from build123d import *

# Parameters (mm, degrees)
SKETCH1_W                                            = 150
SKETCH1_H                                            = 300
BOSS_EXTRUDE1_DEPTH                                  = 20
SKETCH2_W                                            = 150
SKETCH2_H                                            = 8
BOSS_EXTRUDE2_DEPTH                                  = 3
CBORE_FOR_M6_HEX_SOCKET_THIN_HEAD_CAP_SC_D           = 6.6
CBORE_FOR_M6_HEX_SOCKET_THIN_HEAD_CAP_SC_DEPTH       = 24.5
CBORE_FOR_M6_HEX_SOCKET_THIN_HEAD_CAP_SC_CBORE_D     = 11
CBORE_FOR_M6_HEX_SOCKET_THIN_HEAD_CAP_SC_CBORE_DEPTH = 4.5
M8_TAPPED_HOLE1_D                                    = 6.8
M8_TAPPED_HOLE1_DEPTH                                = 33.75
FILLET1_R                                            = 2.5


with BuildPart() as part:
    # Sketch1 → Boss-Extrude1 (new body)
    with BuildSketch(Plane(origin=(0, 0, 0), x_dir=(1, 0, 0), z_dir=(0, 1, 0))):
        Rectangle(SKETCH1_W, SKETCH1_H)
    extrude(amount=BOSS_EXTRUDE1_DEPTH)

    # Sketch2 → Boss-Extrude2 (add)
    with BuildSketch(Plane(origin=(0, 0, 0), x_dir=(1, 0, 0), z_dir=(0, 1, 0))):
        with Locations((0, -130)):
            Rectangle(SKETCH2_W, SKETCH2_H)
        with Locations((0, 130)):
            Rectangle(SKETCH2_W, SKETCH2_H)
    extrude(amount=-BOSS_EXTRUDE2_DEPTH)

    # CBORE for M6 Hex Socket Thin Head Cap Screw1
    with Locations(Plane(origin=(0, 20, 0), x_dir=(1, 0, 0), z_dir=(0, 1, 0))):
        with Locations((0, -130), (0, 130)):
            CounterBoreHole(CBORE_FOR_M6_HEX_SOCKET_THIN_HEAD_CAP_SC_D / 2, CBORE_FOR_M6_HEX_SOCKET_THIN_HEAD_CAP_SC_CBORE_D / 2, CBORE_FOR_M6_HEX_SOCKET_THIN_HEAD_CAP_SC_CBORE_DEPTH, depth=CBORE_FOR_M6_HEX_SOCKET_THIN_HEAD_CAP_SC_DEPTH)

    # M8 Tapped Hole1
    with Locations(Plane.ZY.offset(75)):
        with Locations((0, 10)):
            Hole(M8_TAPPED_HOLE1_D / 2, depth=M8_TAPPED_HOLE1_DEPTH)

    # Fillet1
    fillet1_edges = [part.edges().sort_by_distance(p)[0] for p in [
        (-75, 10, -150),
        (75, 10, -150),
        (75, 10, 150),
        (-75, 10, 150),
    ]]
    fillet(fillet1_edges, radius=FILLET1_R)


solid = part.part
Geometry check sheet. Reference: the model listing, model coordinates, mm. A direction names the side the tool comes from. Give positions to 0.01 mm unless a question says otherwise; leave off trailing zeros. Order: outer loops, then holes, each group sorted by start corner. A loop starts at its lowest first (then second) coordinate and runs counter-clockwise, first axis right, second up. Notation, with made-up numbers: (14.5, -2.5) - (69.5, -2.5) arc R20 ccw to (69.5, 27.5) - close; hole circle Ø2 at (11.5, 85). An arc over 180 degrees is marked (long way). Answer as a JSON object with one key per item and string values.
(1) Cross-section at B-B (z = 130). Record the cut outline in (x, y), then the cut area to 3 significant figures.
Report:
{"outline": "(-75, -3) - (-3.3, -3) - (-3.3, 15.5) - (-5.5, 15.5) - (-5.5, 20) - (-75, 20) - close; (3.3, -3) - (75, -3) - (75, 20) - (5.5, 20) - (5.5, 15.5) - (3.3, 15.5) - close", "area": "3,280 mm^2"}
(2) Cross-section at D-D (z = -36.5). Record the cut outline in (x, y).
Report:
{"outline": "(-75, 0) - (75, 0) - (75, 20) - (-75, 20) - close"}
(3) Depth check by flat-ended pin: pin 1 Ø5 at (x, z) = (-59.5, -109) entering from -Y; pin 2 Ø0.9 at (x, y) = (33.5, -1) entering from -Z; pin 3 Ø2 at (y, z) = (10, -0.5) entering from -X. Enter the tip coordinate at first touch or a pass-through.
Report:
{"pin 1": "y = 0", "pin 2": "z = -134", "pin 3": "x = -41.25"}
(4) Material ranges on line 1 (Z direction, x = 0, y = 6.5); line 2 (Y direction, x = -59, z = 0); line 3 (X direction, y = 18.15, z = 130), recorded low to high.
Report:
{"line 1": "-150 to -133.3, -126.7 to 126.7, 133.3 to 150", "line 2": "0 to 6.6, 13.4 to 20", "line 3": "-75 to -5.5, 5.5 to 75"}
(5) Tool access check on faces 5 (the flat face through (-1, 0, -2)), 6 (the flat face through (-1, 0, -142)), 7 (the flat face through (-1, 0, 142)), 8 (the flat face through (0, 15.5, 134)), 9 (the cylindrical face through (-57.89, 6.68, 0.74)). Record the directions out of +Z, -Z, +X, -X, +Y, -Y that give a thin tool (end or side, any length) a straight path to the whole face; none if there is none.
Report:
{"face 5": "+X, -X, -Y", "face 6": "-Z, +X, -X, -Y", "face 7": "+Z, +X, -X, -Y", "face 8": "+Y", "face 9": "-X"}
(6) Cross-section at C-C (z = 0). Record the cut outline in (x, y).
Report:
{"outline": "(-75, 0) - (75, 0) - (75, 20) - (-75, 20) - (-75, 13.4) - (-41.25, 13.4) - (-41.25, 6.6) - (-75, 6.6) - close"}
(7) Draft check along X on faces 1 (the flat face through (-41.25, 10, 0)), 2 (the flat face through (-1, 10, -150)), 3 (the cylindrical face through (-0.716, 17.782, 124.547)), 4 (the cylindrical face through (-0.716, 17.782, -135.453)). Enter one of: released by +X, released by -X, zero draft, split by the parting line, or undercut.
Report:
{"face 1": "released by -X", "face 2": "zero draft", "face 3": "undercut", "face 4": "undercut"}
(8) Cross-section at A-A (x = 0). Record the cut outline in (y, z), then the cut area to 3 significant figures.
Report:
{"outline": "(-3, -134) - (0, -134) - (0, -150) - (20, -150) - (20, -135.5) - (15.5, -135.5) - (15.5, -133.3) - (-3, -133.3) - close; (-3, -126.7) - (15.5, -126.7) - (15.5, -124.5) - (20, -124.5) - (20, 124.5) - (15.5, 124.5) - (15.5, 126.7) - (-3, 126.7) - (-3, 126) - (0, 126) - (0, -126) - (-3, -126) - close; (-3, 133.3) - (15.5, 133.3) - (15.5, 135.5) - (20, 135.5) - (20, 150) - (0, 150) - (0, 134) - (-3, 134) - close", "area": "5,700 mm^2"}
